The listing builds one solid part. Answer for the finished solid, in the listing's coordinates (mm). Face numbers are marked on the shaded views. A direction names the side the tool comes from. Coordinates: 2 decimals unless noted, no trailing zeros. Order: outer loops, then holes, each group sorted by start corner. A loop starts at its lowest first (then second) coordinate and runs counter-clockwise, first axis right, second up.
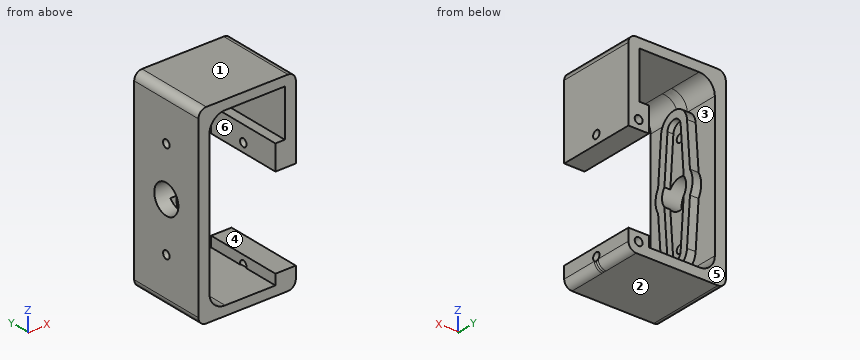
Autodesk Inventor part; units mm, degrees
ref_plane "YZ Plane" through (0, 0, 0) normal (1, 0, 0) x (0, 1, 0)
ref_plane "XZ Plane" through (0, 0, 0) normal (0, 1, 0) x (-1, 0, 0)
ref_plane "XY Plane" through (0, 0, 0) normal (0, 0, 1) x (1, 0, 0)
sketch "スケッチ1" plane through (0, 0, 0) normal (0, 1, 0) x (-1, 0, 0)
  line L0 (34.0614, 0) -> (-44.6235, 0)
  line L1 (0, 24.4) -> (0, -24.4)
  line L2 (0, -24.4) -> (-24.8, -24.4)
  line L3 (-24.8, -24.4) -> (-24.8, -22)
  line L4 (-24.8, -22) -> (-2.8, -22)
  line L5 (-2.8, -22) -> (-2.8, 22)
  line L6 (-2.8, 22) -> (-24.8, 22)
  line L7 (-24.8, 22) -> (-24.8, 24.4)
  line L8 (-24.8, 24.4) -> (0, 24.4)
  point P0 (0, 0)
  dimension "d0" = 2.8
  dimension "d1" = 48.8
  dimension "d2" = 24.4
  dimension "d3" = 2.4
  dimension "d4" = 2.4
  dimension "d5" = 22
extrude "押し出し1" add sketch "スケッチ1" along normal blind 20
sketch "スケッチ2" plane through (2.8, 0, 22) normal (1, 0, 0) x (0, 0, -1)
  line L0 (0, 20) -> (44, 20)
  line L1 (22, 20) -> (22, 0)
  line L2 (0, 0) -> (44, 0)
  line L3 (-2.4, 0) -> (-2.4, 20)
  line L4 (-2.4, 10) -> (46.4, 10)
  line L5 (46.4, 0) -> (46.4, 20)
  circle A0 centre (22, 10) radius 3.75
  arc A1 (7.6386, 12.0436) -> (7.6386, 7.9564) centre (7.8, 10) ccw
  line L6 (19.75, 13) -> (7.6386, 12.0436)
  line L7 (19.75, 7) -> (7.6386, 7.9564)
  circle A2 centre (9.5, 10) radius 1
  arc A3 (36.3614, 7.9564) -> (36.3614, 12.0436) centre (36.2, 10) ccw
  line L8 (24.25, 13) -> (36.3614, 12.0436)
  line L9 (24.25, 7) -> (36.3614, 7.9564)
  circle A4 centre (34.5, 10) radius 1
  line L10 (19.0799, 14.9533) -> (7.4812, 14.0374)
  arc A5 (7.4812, 14.0374) -> (7.4812, 5.9626) centre (7.8, 10) ccw
  line L11 (7.4812, 5.9626) -> (19.0799, 5.0467)
  circle A6 centre (22, 10) radius 5.75
  line L12 (24.9201, 14.9533) -> (36.5188, 14.0374)
  arc A7 (36.5188, 5.9626) -> (36.5188, 14.0374) centre (36.2, 10) ccw
  line L13 (36.5188, 5.9626) -> (24.9201, 5.0467)
  point P0 (18.25, 10)
  point P1 (22, 6.25)
  point P2 (24.25, 13)
  point P3 (24.25, 7)
  point P4 (19.75, 7)
  point P5 (27.0332, 12.7802)
  point P6 (27.0332, 7.2198)
  point P7 (16.9668, 12.7802)
  point P8 (16.9668, 7.2198)
  dimension "d9" = 7.5
  dimension "d8" = 24.4
  dimension "d10" = 6
  dimension "d11" = 14.2
  dimension "d12" = 2.05
  dimension "d13" = 2
  dimension "d14" = 12.5
  dimension "d34" = 2
  dimension "d35" = 2
  dimension "d36" = 2
extrude "押し出し2" cut sketch "スケッチ2" against normal through all contours A0 L4 L1 | L1 L4 A0 | L4 A0 L1 | L1 A0 L4 | A4 L4 | L4 A4 | A2 L4 | L4 A2
extrude "押し出し6" add sketch "スケッチ2" along normal blind 2.2 contours A6 L8 A0 L1 | L1 A0 L6 A6 | L12 A7 L4 A3 L8 A6 | A6 L6 A1 L4 A5 L10 | A0 L9 A6 L1 | L1 A6 L7 A0 | A7 L13 A6 L9 A3 L4 | L4 A1 L7 A6 L11 A5
extrude "押し出し3" add sketch "スケッチ2" along normal blind 0.7 contours L8 A6 L4 A0 | A0 L4 A6 L6 | L8 A3 L4 A4 A6 | A6 L4 A2 A1 L6 | A0 L7 A6 L4 | L4 A6 L9 A0 | L4 A4 A3 L9 A6 | A6 L7 A1 L4 A2
sketch "スケッチ3" plane through (24.8, 0, -22) normal (1, 0, 0) x (0, 0, -1)
  line L0 (-46.4, 0) -> (-46.4, 20)
  line L1 (2.4, 0) -> (-46.4, 0)
  line L2 (-46.4, 20) -> (-25.65, 20)
  line L3 (-25.65, 20) -> (-25.65, 0)
  line L4 (-25.65, 0) -> (-46.4, 0)
  line L5 (-46.4, 0) -> (-46.4, 20)
  line L6 (2.4, 20) -> (-46.4, 20)
  line L7 (2.4, 20) -> (-2.65, 20)
  line L8 (-2.65, 20) -> (-2.65, 0)
  line L9 (-2.65, 0) -> (2.4, 0)
  line L10 (2.4, 0) -> (2.4, 20)
  line L11 (-46.4, 10) -> (2.4, 10)
  line L12 (-19.4, 20) -> (-19.4, 0)
  circle A0 centre (-27.9, 10) radius 1
  circle A1 centre (-0.4, 10) radius 1
  point P0 (-22, 0)
  point P1 (-2.65, 20)
  point P2 (-2.65, 0)
  point P3 (2.4, 0)
  dimension "d19" = 27
  dimension "d20" = 6.25
  dimension "d21" = 16.75
  dimension "d22" = 2.25
  dimension "d23" = 2.25
  dimension "d24" = 2
extrude "押し出し4" add sketch "スケッチ3" against normal blind 5.2 contours L0 L11 A0 L3 L1 | L0 L2 L3 L11 A0 | L8 L11 A1 L10 L1 | L8 L6 L10 L11 A1
extrude "押し出し8" cut sketch "スケッチ3" against normal blind 5 contours A1 L11 | L11 A1
sketch "スケッチ4" plane through (0, 20, 0) normal (0, 1, 0) x (1, 0, 0)
  line L0 (22.2, 20.9661) -> (22.2, -25.0757)
  line L1 (19.6, -22) -> (19.6, -3.65)
  circle A0 centre (22.2, -5.9) radius 1
  circle A1 centre (22.2, 21.6) radius 1
  line L2 (24.8, -3.65) -> (19.6, -3.65)
  line L3 (24.8, 19.35) -> (19.6, 19.35)
  line L4 (24.8, -24.4) -> (24.8, -3.65)
  point P0 (0, 0)
  point P1 (24.8, -24)
  dimension "d28" = 2.6
  dimension "d29" = 2.25
  dimension "d30" = 2
  dimension "d31" = 2.25
extrude "押し出し5" cut sketch "スケッチ4" against normal blind 7
sketch "スケッチ5" plane through (0, 20, 0) normal (0, 1, 0) x (1, 0, 0)
  line L0 (19.6, -22) -> (2.8, -22)
  line L1 (19.6, -22) -> (22, -22)
  line L2 (22, -22) -> (22, -10)
  line L3 (22, -10) -> (19.6, -10)
  line L4 (19.6, -22) -> (19.6, -3.65)
  line L5 (24.8, -24.4) -> (24.8, -3.65)
  point P0 (0, 0)
  dimension "d39" = 2.8
  dimension "d40" = 12
extrude "押し出し7" cut sketch "スケッチ5" against normal through all
fillet "フィレット2" radius 2 2 edges at (0, 10, 24.4) (0, 10, -24.4)
fillet "フィレット4" radius 2 2 edges at (24.8, 10, 24.4) (24.8, 10, -24.4)
fillet "フィレット5" radius 4 1 edges at (2.8, 10, -22)
fillet "フィレット6" radius 4 1 edges at (2.8, 10, 22)
properties part number "joint4"
(1) Find section D-D on y = 3.25. Determine the outline of the cut face in (x, z), then the cut area to 3 significant figures.
(2) Find section A-A on x = 8. Determine the outline of the cut face in (y, z), then the cut area to 3 significant figures.
(3) Find section B-B on z = -12.5. Determine the outline of the cut face in (x, y), then the cut area to 3 significant figures.
(4) The mould has two halves that part along Z. Classify the marked faces 1, 2 and 3: pulls with the +Z half, pulls with the -Z half, needs draft (parallel to the pull), parting line crosses it, or undercut.
(5) Given pin 1 Ø2.5 at (y, z) = (4.5, -2) entering from +X; pin 2 Ø1.8 at (x, z) = (22.2, -21.6) entering from +Y; pin 3 Ø1.5 at (y, z) = (17, -6) entering from +X, each flat-ended and moving along its own axis, determine where each tip first touches the part or whether it passes through.
(6) Find the intervals of material crossed by probe 1 along X at (y, z) = (17, 5.9); probe 2 along Z at (x, y) = (21.45, 10); probe 3 along Z at (x, y) = (22.2, 14.75), in increasing order.
(7) Find section C-C on z = 12.5. Determine the outline of the cut face in (x, y).
(8) A tool of negligible diameter and unlimited length cuts with its end or side. For the marked faces 4, 5 and 6, from which of +Z, -Z, +X, -X, +Y, -Y can it reach the whole face along a straight path? Write none if from no direction.
Resolved:
1. outline: (0, -22.4) arc R2 ccw to (2, -24.4) - (22.8, -24.4) arc R2 ccw to (24.8, -22.4) - (24.8, -19.35) - (19.6, -19.35) - (19.6, -22) - (6.8, -22) arc R4 cw to (2.8, -18) - (2.8, 18) arc R4 cw to (6.8, 22) - (22, 22) - (22, 10) - (19.6, 10) - (19.6, 3.65) - (24.8, 3.65) - (24.8, 22.4) arc R2 ccw to (22.8, 24.4) - (2, 24.4) arc R2 ccw to (0, 22.4) - close
1. area: 326 mm2
2. outline: (0, -24.4) - (20, -24.4) - (20, -22) - (0, -22) - close; (0, 22) - (20, 22) - (20, 24.4) - (0, 24.4) - close
2. area: 96.0 mm2
3. outline: (0, 0) - (2.8, 0) - (2.8, 5.8) - (5, 5.8) - (5, 7.81) - (3.5, 7.81) - (3.5, 9) - (0, 9) - close; (0, 11) - (3.5, 11) - (3.5, 12.19) - (5, 12.19) - (5, 14.2) - (2.8, 14.2) - (2.8, 20) - (0, 20) - close
3. area: 60.9 mm2
4. face 1: pulls with the +Z half
4. face 2: pulls with the -Z half
4. face 3: undercut
5. pin 1: stops at x = 5
5. pin 2: stops at y = 13
5. pin 3: stops at x = 2.8
6. probe 1: x = 0 to 2.8, 19.6 to 21.2, 23.2 to 24.8
6. probe 2: z = -24.4 to -22.6, -20.6 to -19.35, 3.65 to 4.9, 6.9 to 10, 22 to 24.4
6. probe 3: z = -24.4 to -22.6, -20.6 to -19.35, 3.65 to 4.9, 6.9 to 24.4
7. outline: (0, 0) - (2.8, 0) - (2.8, 5.8) - (5, 5.8) - (5, 7.81) - (3.5, 7.81) - (3.5, 9) - (0, 9) - close; (0, 11) - (3.5, 11) - (3.5, 12.19) - (5, 12.19) - (5, 14.2) - (2.8, 14.2) - (2.8, 20) - (0, 20) - close; (22, 0) - (24.8, 0) - (24.8, 20) - (22, 20) - close
8. face 4: +X, +Y, -Y
8. face 5: +Z, -Z, +X, -X, +Y
8. face 6: +Y, -Y
